from build123d import *

# Parameters (mm, degrees)
SKETCH1_R           = 1.6
BOSS_EXTRUDE1_DEPTH = 3
SKETCH3_R           = 2.6
SKETCH3_R_2         = 1.6
CUT_EXTRUDE2_DEPTH  = 3
FILLET2_R           = 10


with BuildPart() as part:
    # Sketch1 → Boss-Extrude1 (new body)
    with BuildSketch(Plane(origin=(0, 0, 0), x_dir=(1, 0, 0), z_dir=(0, 1, 0))):
        with BuildLine():
            Line((0, 0), (0, 95))
            Line((0, 95), (40, 95))
            Line((40, 95), (40, 0))
            ThreePointArc((40, 0), (20, -20), (0, 0))
        make_face()
        with Locations(Location((20, 0, 0), (0, 0, 270))):
            Circle(SKETCH1_R, mode=Mode.SUBTRACT)
    extrude(amount=BOSS_EXTRUDE1_DEPTH)

    # Sketch3 → Cut-Extrude2 (cut)
    with BuildSketch(Plane(origin=(0, 3, 0), x_dir=(1, 0, 0), z_dir=(0, 1, 0))):
        with Locations(Location((10, 85, 0), (0, 0, 270))):
            Circle(SKETCH3_R)
        with Locations(Location((30, 85, 0), (0, 0, 270))):
            Circle(SKETCH3_R)
        with Locations(Location((10, 35, 0), (0, 0, 270))):
            Circle(SKETCH3_R_2)
        with Locations(Location((30, 35, 0), (0, 0, 270))):
            Circle(SKETCH3_R_2)
    extrude(amount=-CUT_EXTRUDE2_DEPTH, mode=Mode.SUBTRACT)

    # Fillet2
    fillet2_edges = [part.edges().sort_by_distance(p)[0] for p in [
        (0, 1.5, -95),
        (40, 1.5, -95),
    ]]
    fillet(fillet2_edges, radius=FILLET2_R)


solid = part.part
Can you work these out from the model? Positions are in its coordinate system, mm. Round coordinates to 2 decimals unless told otherwise and drop trailing zeros. Order: outer loops, then holes, each group sorted by start corner. A loop starts at its lowest first (then second) coordinate and runs counter-clockwise, first axis right, second up. Notation, with made-up numbers: M 9.25,21 L 61.25,21 A33 cw 61.25,60 Z; hole C 4,-6 d6. An arc over 180 degrees is marked long. Use a Markdown table: item, result.
1) Imagine slicing it at C-C (z = -35). List the corners of the cut face in (x, y) for me.
Geometry says:
| item | result |
|---|---|
| outline | M 0,0 L 8.4,0 L 8.4,3 L 0,3 Z; M 11.6,0 L 28.4,0 L 28.4,3 L 11.6,3 Z; M 31.6,0 L 40,0 L 40,3 L 31.6,3 Z |
2) Imagine slicing it at A-A (y = 2.45). List the corners of the cut face in (x, z) for me, then the cut area to 3 significant figures.
Geometry says:
| item | result |
|---|---|
| outline | M 0,-85 A10 ccw 10,-95 L 30,-95 A10 ccw 40,-85 L 40,0 A20 ccw 0,0 Z; hole C 10,-85 d5.2; hole C 10,-35 d3.2; hole C 20,0 d3.2; hole C 30,-85 d5.2; hole C 30,-35 d3.2 |
| area | 4,320 mm² |
3) I'm going to push a flat-ended pin straight in: P1, Ø3.5, axis at x = 10, z = -35, coming from the +Y side. Where does the tip first touch, or does it pass through?
Geometry says:
| item | result |
|---|---|
| P1 | stops at y = 3 |
4) Imagine slicing it at D-D (z = 12.5). List the corners of the cut face in (x, y) for me, then the cut area to 3 significant figures.
Geometry says:
| item | result |
|---|---|
| outline | M 4.39,0 L 35.61,0 L 35.61,3 L 4.39,3 Z |
| area | 93.7 mm² |
5) Imagine slicing it at B-B (x = 20). List the corners of the cut face in (y, z) for me, then the cut area to 3 significant figures.
Geometry says:
| item | result |
|---|---|
| outline | M 0,-95 L 3,-95 L 3,-1.6 L 0,-1.6 Z; M 0,1.6 L 3,1.6 L 3,20 L 0,20 Z |
| area | 335 mm² |
6) If I drill on line 1 along X through (y, z) = (2.05, -35); line 2 along Z through (x, y) = (32, 0.85); line 3 along X through (y, z) = (2.2, 1), over which ranges is the centre line in solid material (lowest first)?
Geometry says:
| item | result |
|---|---|
| line 1 | x = 0 to 8.4, 11.6 to 28.4, 31.6 to 40 |
| line 2 | z = -94.8 to -86.66, -83.34 to 16 |
| line 3 | x = 0.03 to 18.75, 21.25 to 39.97 |
7) If we mould it in two halves opening along X, with no side actions, what happens to faces 1 (the face through (20, 3, -38)), 2 (the face through (31.586, 1.521, -35.208)), 3 (the face through (20, 1, 20)), 4 (the face through (21.586, 1.479, -0.208))? For each: +X half, -X half, draft (parallel to the pull), parting line (faces both ways), or undercut.
Geometry says:
| item | result |
|---|---|
| face 1 | draft |
| face 2 | undercut |
| face 3 | parting line |
| face 4 | undercut |
